from build123d import *

# Parameters (mm, degrees)
F0_W     = 76.2
F0_H     = 76.2
F1_DEPTH = 3.175
F4_DEPTH = 76.2
F5_DEPTH = 76.2
F6_R     = 1.5875
F7_DEPTH = 3.176


with BuildPart() as f1:
    # F0 (on Top) → F1 (new body)
    with BuildSketch(Plane.XY):
        Rectangle(F0_W, F0_H)
    extrude(amount=F1_DEPTH)

    # F3 (on face) → F4 (cut)
    with BuildSketch(Plane(origin=(0, 38.1, 0), x_dir=(-1, 0, 0), z_dir=(0, 1, 0))):
        Polygon((-38.1, 3.175), (-38.1, 0), (-34.925, 3.175), align=None)
        Polygon((34.925, 3.175), (38.1, 0), (38.1, 3.175), align=None)
    extrude(amount=-F4_DEPTH, mode=Mode.SUBTRACT)

    # F2 (on face) → F5 (cut)
    with BuildSketch(Plane.YZ.offset(38.1)):
        Polygon((34.925, 3.175), (38.1, 0), (38.1, 3.175), align=None)
        Polygon((-38.1, 3.175), (-38.1, 0), (-34.925, 3.175), align=None)
    extrude(amount=-F5_DEPTH, mode=Mode.SUBTRACT)

    # F6 (on face) → F7 (cut, through all)
    with BuildSketch(Plane(origin=(0, 0, 0), x_dir=(1, 0, 0), z_dir=(0, 0, -1))):
        with Locations((-25.4, 25.4)):
            Circle(F6_R)
        with Locations((-12.7, 25.4)):
            Circle(F6_R)
        with Locations((12.7, 25.4)):
            Circle(F6_R)
        with Locations((25.4, 25.4)):
            Circle(F6_R)
        with Locations((0, 25.4)):
            Circle(F6_R)
        with Locations((0, 12.7)):
            Circle(F6_R)
        with Locations((-12.7, 12.7)):
            Circle(F6_R)
        with Locations((-25.4, 12.7)):
            Circle(F6_R)
        with Locations((-25.4, 0)):
            Circle(F6_R)
        with Locations((-12.7, 0)):
            Circle(F6_R)
        Circle(F6_R)
        with Locations((12.7, 12.7)):
            Circle(F6_R)
        with Locations((25.4, 12.7)):
            Circle(F6_R)
        with Locations((25.4, 0)):
            Circle(F6_R)
        with Locations((12.7, 0)):
            Circle(F6_R)
        with Locations((-25.4, -12.7)):
            Circle(F6_R)
        with Locations((-25.4, -25.4)):
            Circle(F6_R)
        with Locations((-12.7, -25.4)):
            Circle(F6_R)
        with Locations((0, -25.4)):
            Circle(F6_R)
        with Locations((12.7, -25.4)):
            Circle(F6_R)
        with Locations((25.4, -25.4)):
            Circle(F6_R)
        with Locations((25.4, -12.7)):
            Circle(F6_R)
        with Locations((12.7, -12.7)):
            Circle(F6_R)
        with Locations((0, -12.7)):
            Circle(F6_R)
        with Locations((-12.7, -12.7)):
            Circle(F6_R)
    extrude(amount=-F7_DEPTH, mode=Mode.SUBTRACT)


solid = f1.part
Geometry check sheet. Reference: the model listing, model coordinates, mm. Give positions to 0.01 mm unless a question says otherwise; leave off trailing zeros. Loops run counter-clockwise (first coordinate to the right, second up) from the corner with the lowest first, then second, coordinate; pieces in that order, holes last.
(1) Section check A-A on z = 2.25. Count the separate pieces of the cut face and the enclosed holes in it, then the cut area to 3 significant figures.
From the geometry:
separate pieces: 1
enclosed holes: 25
area: 4,940 mm2
(2) Release check for a two-part mould opening along Y. For faces 1 (the cylindrical face through (14.214, -0.477, 1.565)), 2 (the flat face through (0.5, 36.5, 1.6)), 3 (the flat face through (8, 1, 0)) record: released by +Y, released by -Y, zero draft, split by the parting line, or undercut.
From the geometry:
face 1: undercut
face 2: released by +Y
face 3: zero draft
(3) Section check B-B on y = 12.7. Record the cut outline in (x, z) (1 decimal).
From the geometry:
outline: (-38.1, 0) - (-27, 0) - (-27, 3.2) - (-34.9, 3.2) - close; (-23.8, 0) - (-14.3, 0) - (-14.3, 3.2) - (-23.8, 3.2) - close; (-11.1, 0) - (-1.6, 0) - (-1.6, 3.2) - (-11.1, 3.2) - close; (1.6, 0) - (11.1, 0) - (11.1, 3.2) - (1.6, 3.2) - close; (14.3, 0) - (23.8, 0) - (23.8, 3.2) - (14.3, 3.2) - close; (27, 0) - (38.1, 0) - (34.9, 3.2) - (27, 3.2) - close
(4) Depth check by flat-ended pin: pin 1 Ø4 at (x, y) = (25.4, -12.7) entering from +Z (3 decimals); pin 2 Ø3 at (x, y) = (0, 25.4) entering from +Z; pin 3 Ø1 at (y, z) = (13, 2) entering from +X. Enter the tip coordinate at first touch or a pass-through.
From the geometry:
pin 1: stops at z = 3.175
pin 2: passes through
pin 3: stops at x = 36.6
(5) Section check D-D on x = 18.5. Record the cut outline in (y, z) (3 decimals), then the cut area to 3 significant figures.
From the geometry:
outline: (-38.1, 0) - (38.1, 0) - (34.925, 3.175) - (-34.925, 3.175) - close
area: 232 mm2
(6) Thickness scan on L1, parallel to X at y = 0, z = 1.35; L2, parallel to Y at x = 13, z = 2.5; L3, parallel to Y at x = 12.7, z = 1.15. Record the ranges inside material, lowest first.
From the geometry:
L1: x = -36.75 to -26.99, -23.81 to -14.29, -11.11 to -1.59, 1.59 to 11.11, 14.29 to 23.81, 26.99 to 36.75
L2: y = -35.6 to -26.96, -23.84 to -14.26, -11.14 to -1.56, 1.56 to 11.14, 14.26 to 23.84, 26.96 to 35.6
L3: y = -36.95 to -26.99, -23.81 to -14.29, -11.11 to -1.59, 1.59 to 11.11, 14.29 to 23.81, 26.99 to 36.95
